Autodesk Inventor part; units mm, degrees
ref_plane "YZ Plane" through (0, 0, 0) normal (1, 0, 0) x (0, 1, 0)
ref_plane "XZ Plane" through (0, 0, 0) normal (0, 1, 0) x (-1, 0, 0)
ref_plane "XY Plane" through (0, 0, 0) normal (0, 0, 1) x (1, 0, 0)
sketch "Esboço1" plane through (0, 0, 0) normal (0, 0, 1) x (1, 0, 0)
  circle A0 centre (0, 0) radius 9.5
  dimension "d0" = 19
extrude "Extrusão1" add sketch "Esboço1" along normal blind 25
sketch "Esboço4" plane through (0, 0, 25) normal (0, 0, 1) x (1, 0, 0)
  circle A0 centre (0, 0) radius 1.7116
hole "Furo1" at (0, 0, 25) direction (0, 0, -1) diameter 5 end through all counterbore diameter 8 counterbore depth 9.5
fillet "Arredondamento1" radius 1 2 edges at (-9.5, 0, 0) (-9.5, 0, 25)
properties part number "Acoplamento5Para8"
Geometry check sheet. Reference: the model listing, model coordinates, mm. A direction names the side the tool comes from. Round coordinates to 2 decimals unless told otherwise and drop trailing zeros. Loops run counter-clockwise (first coordinate to the right, second up) from the corner with the lowest first, then second, coordinate; pieces in that order, holes last. Notation, with made-up numbers: (24, 80) -> (74, 80) arc R11 ccw to (74, 92) -> close; hole circle Ø5 at (2.5, 20). An arc over 180 degrees is marked (long way). Answer as a JSON object with one key per item and string values. Group by question number.
Item 1: Set-up check for faces 1 (the face through (-2, -2, 15.5)), 2 (the face through (2, -2, 0)): record each of +Z, -Z, +X, -X, +Y, -Y from which the full face is reachable in a straight line by a thin tool's end or side.
Item 2: Thickness scan on line 1 along Y through (x, z) = (0, 6.25); line 2 along Y through (x, z) = (0, 21.25); line 3 along X through (y, z) = (1, 15). Record the ranges inside material, lowest first.
Item 3: Depth check by flat-ended pin: pin 1 Ø3 at (x, y) = (0, 0) entering from +Z; pin 2 Ø1.5 at (y, z) = (-4.5, 11) entering from -X; pin 3 Ø5 at (y, z) = (6, 17) entering from +X; pin 4 Ø1 at (y, z) = (-5.5, 14) entering from -X. Enter the tip coordinate at first touch or a pass-through.
Item 4: Cross-section at D-D, the plane z = 18.75. Record the cut outline in (x, y).
Item 5: Cross-section at C-C, the plane z = 2.5. Record the cut outline in (x, y).
Item 6: Cross-section at A-A, the plane y = 0. Record the cut outline in (x, z).
Item 7: Release check for a two-part mould opening along X. For faces 3 (the face through (4, -2, 25)), 4 (the face through (3.905, 0.867, 20.184)), 5 (the face through (4.38, 8.43, 12.34)), 6 (the face through (2.44, 0.54, 7.64)) record: pulls with the +X half, pulls with the -X half, needs draft (parallel to the pull), parting line crosses it, or undercut.
Determined:
{
 "1": {"face 1": "+Z", "face 2": "-Z, +X, -X, +Y, -Y"},
 "2": {"line 1": "y = -9.5 to -2.5, 2.5 to 9.5", "line 2": "y = -9.5 to -4, 4 to 9.5", "line 3": "x = -9.45 to -2.29, 2.29 to 9.45"},
 "3": {"pin 1": "passes through", "pin 2": "stops at x = -8.73", "pin 3": "stops at x = 8.83", "pin 4": "stops at x = -8.08"},
 "4": {"outline": "circle Ø19 at (0, 0); hole circle Ø8 at (0, 0)"},
 "5": {"outline": "circle Ø19 at (0, 0); hole circle Ø5 at (0, 0)"},
 "6": {"outline": "(-9.5, 1) arc R1 ccw to (-8.5, 0) -> (-2.5, 0) -> (-2.5, 15.5) -> (-4, 15.5) -> (-4, 25) -> (-8.5, 25) arc R1 ccw to (-9.5, 24) -> close; (2.5, 0) -> (8.5, 0) arc R1 ccw to (9.5, 1) -> (9.5, 24) arc R1 ccw to (8.5, 25) -> (4, 25) -> (4, 15.5) -> (2.5, 15.5) -> close"},
 "7": {"face 3": "needs draft", "face 4": "undercut", "face 5": "parting line crosses it", "face 6": "undercut"}
}
